```python
from build123d import *

# Parameters (mm, degrees)
SKETCH_1_W                   = 300
SKETCH_1_H                   = 15
EXTRUDE_328_DEPTH            = 15
HOLE_WIZARD_M6_D             = 5
HOLE_WIZARD_M6_CSINK_D       = 12.6
HOLE_WIZARD_M6_CSINK_ANGLE   = 90
HOLE_WIZARD_8_1_D            = 8.1
SKETCH_8_W                   = 250
SKETCH_8_H                   = 15
EXTRUDE_2374_DEPTH           = 5.4
SKETCH_9_R                   = 4
CUT_EXTRUDE_2694_DEPTH       = 1.5
SKETCH_10_W                  = 100
SKETCH_10_H                  = 15
CUT_EXTRUDE_2982_DEPTH       = 5.4
HOLE_WIZARD_1_M6_D           = 5
HOLE_WIZARD_1_M6_CSINK_D     = 12.6
HOLE_WIZARD_1_M6_CSINK_ANGLE = 90
HOLE_WIZARD_2_M6_D           = 5
HOLE_WIZARD_2_M6_CSINK_D     = 12.6
HOLE_WIZARD_2_M6_CSINK_ANGLE = 90
CHAMFER_1_SIZE               = 5
CHAMFER_2_SIZE               = 1


with BuildPart() as part:
    # Эскиз1 → Extrude 328 (new body)
    with BuildSketch(Plane(origin=(0, 0, 0), x_dir=(1, 0, 0), z_dir=(0, 1, 0))):
        Rectangle(SKETCH_1_W, SKETCH_1_H)
    extrude(amount=EXTRUDE_328_DEPTH)

    # Крепление шарнира M6 (through all)
    with Locations(Plane(origin=(0, 15, 0), x_dir=(1, 0, 0), z_dir=(0, 1, 0))):
        with Locations((-115, 0), (115, 0)):
            CounterSinkHole(HOLE_WIZARD_M6_D / 2, HOLE_WIZARD_M6_CSINK_D / 2, counter_sink_angle=HOLE_WIZARD_M6_CSINK_ANGLE)

    # Отверстие-8.1мм (through all)
    with Locations(Plane(origin=(0, 15, 0), x_dir=(1, 0, 0), z_dir=(0, 1, 0))):
        with Locations((-140, 0), (140, 0)):
            Hole(HOLE_WIZARD_8_1_D / 2)

    # Эскиз8 → Extrude 2374 (add)
    with BuildSketch(Plane.XY.offset(7.5)):
        with Locations((0, 7.5)):
            Rectangle(SKETCH_8_W, SKETCH_8_H)
    extrude(amount=EXTRUDE_2374_DEPTH)

    # Эскиз9 → Cut-Extrude 2694 (cut)
    with BuildSketch(Plane.XY.offset(12.9)):
        with Locations((-105, 7.5)):
            Circle(SKETCH_9_R)
        with Locations((105, 7.5)):
            Circle(SKETCH_9_R)
    extrude(amount=-CUT_EXTRUDE_2694_DEPTH, mode=Mode.SUBTRACT)

    # Эскиз10 → Cut-Extrude 2982 (cut)
    with BuildSketch(Plane.XY.offset(12.9)):
        with Locations((0, 7.5)):
            Rectangle(SKETCH_10_W, SKETCH_10_H)
    extrude(amount=-CUT_EXTRUDE_2982_DEPTH, mode=Mode.SUBTRACT)

    # Прижим-1-M6 (through all)
    with Locations(Plane.XY.offset(12.9)):
        with Locations((-90, 7.5), (90, 7.5)):
            CounterSinkHole(HOLE_WIZARD_1_M6_D / 2, HOLE_WIZARD_1_M6_CSINK_D / 2, counter_sink_angle=HOLE_WIZARD_1_M6_CSINK_ANGLE)

    # Прижим-2-M6 (through all)
    with Locations(Plane.XY.offset(7.5)):
        with Locations((-30, 7.5), (30, 7.5)):
            CounterSinkHole(HOLE_WIZARD_2_M6_D / 2, HOLE_WIZARD_2_M6_CSINK_D / 2, counter_sink_angle=HOLE_WIZARD_2_M6_CSINK_ANGLE)

    # Фаска1
    chamfer_1_edges = [part.edges().sort_by_distance(p)[0] for p in [
        (-150, 7.5, -7.5),
        (150, 7.5, -7.5),
    ]]
    chamfer(chamfer_1_edges, length=CHAMFER_1_SIZE)

    # Фаска2
    chamfer_2_edges = [part.edges().sort_by_distance(p)[0] for p in [
        (-125, 7.5, 12.9),
        (125, 7.5, 12.9),
        (-50, 7.5, 12.9),
        (50, 7.5, 12.9),
    ]]
    chamfer(chamfer_2_edges, length=CHAMFER_2_SIZE)


solid = part.part
```
Here's how the part is built. I have some questions about the finished solid (model axes, mm). A direction names the side the tool comes from. Coordinates: 2 decimals unless noted, no trailing zeros. Order: outer loops, then holes, each group sorted by start corner. A loop starts at its lowest first (then second) coordinate and runs counter-clockwise, first axis right, second up.
1) Imagine slicing it at D-D on x = -104. List the corners of the cut face in (y, z) for me, and give its area (3 significant figures).
2) We'd pull the mould along Z, two halves only. Please class faces 1 (the face through (117.7, 11.4, -0.1)), 2 (the face through (-32.561, 8.306, 3.885)), 3 (the face through (108.695, 5.968, 12.16)): +Z half, -Z half, draft (parallel to the pull), parting line (faces both ways), or undercut.
3) Imagine slicing it at B-B on y = 7.5. State how many separate pieces and enclosed holes the cut face has, and give its area (3 significant figures).
4) Imagine slicing it at A-A on x = 90. List the corners of the cut face in (y, z) for me.
5) I need wall thicknesses on line 1 (Z direction, x = -140, y = 6); line 2 (X direction, y = 8.25, z = -4.25); line 3 (Y direction, x = -30, z = 1.5). Which ranges of each line are inside material? Lowest first, please.
6) Which directions (+Z, -Z, +X, -X, +Y, -Y) give clear straight access to the entire face, cutting with the end or side of a thin tool? Please do faces 4 (the face through (105, 8, 11.4)), 5 (the face through (112.615, 5.522, -0.751)), 6 (the face through (-138, 7, 7.5)).
7) Imagine slicing it at C-C on x = -140. List the corners of the cut face in (y, z) for me.
8) Will these pins go through, and if not, where does the flat tip stop? pin 1 (3.5 mm diameter, centred on y = 11, z = 10, fed in from +X); pin 2 (4.5 mm diameter, centred on x = -135.5, y = 8.5, fed in from +Z); pin 3 (2.5 mm diameter, centred on x = -104.5, y = 7.5, fed in from +Z).
Response values:
1. outline: (0, -7.5) - (15, -7.5) - (15, 12.9) - (11.37, 12.9) - (11.37, 11.4) - (3.63, 11.4) - (3.63, 12.9) - (0, 12.9) - close
1. area: 294 mm2
2. face 1: undercut
2. face 2: +Z half
2. face 3: draft
3. separate pieces: 5
3. enclosed holes: 4
3. area: 4,700 mm2
4. outline: (0, -7.5) - (5, -7.5) - (5, 9.1) - (1.2, 12.9) - (0, 12.9) - close; (10, -7.5) - (15, -7.5) - (15, 12.9) - (13.8, 12.9) - (10, 9.1) - close
5. line 1: z = -7.5 to -4.05, 4.05 to 7.5
5. line 2: x = -148.25 to -92.38, -87.62 to -32.38, -27.62 to 27.62, 32.38 to 87.62, 92.38 to 148.25
5. line 3: y = 0 to 5, 10 to 15
6. face 4: +Z
6. face 5: +Y, -Y
6. face 6: +Z, -X, +Y, -Y
7. outline: (0, -7.5) - (15, -7.5) - (15, -4.05) - (0, -4.05) - close; (0, 4.05) - (15, 4.05) - (15, 7.5) - (0, 7.5) - close
8. pin 1: stops at x = 125
8. pin 2: stops at z = 7.5
8. pin 3: stops at z = 11.4
